Verification items for the finished model (mm, model axes). A direction names the side the tool comes from. Coordinates: 2 decimals unless noted, no trailing zeros. Loops run counter-clockwise (first coordinate to the right, second up) from the corner with the lowest first, then second, coordinate; pieces in that order, holes last.
Q1. Access from +Z, -Z, +X, -X, +Y, -Y to the whole of each face (thin tool, end or side, straight path). Record for faces 1 (the face through (-19.96, 11.57, 17)), 2 (the face through (12.5, 3, 0)).
Q2. Sectioned sample at C-C (y = 42.5). Enter the section's corners in (x, z), then the cut area to 3 significant figures.
Q3. Mould release check, pull along X, two halves, no side actions. Record for faces 3 (the face through (0, 0, 0)), 4 (the face through (-17.5, 45, 0)), 5 (the face through (-22.5, 42, 0)): +X half, -X half, draft (parallel to the pull), parting line (faces both ways), or undercut.
Q4. Sectioned sample at D-D (z = 3). Enter the section's corners in (x, y), then the cut area to 3 significant figures.
Q5. Material ranges on probe 1 along Y at (x, z) = (17.5, 0); probe 2 along Z at (x, y) = (18, 4.5); probe 3 along X at (y, z) = (34.5, 11), recorded low to high.
Q6. Go/stop test with flat-tipped pins: P1, Ø1, axis at x = -15.5, z = -3, coming from the +Y side; P2, Ø2, axis at y = 3.5, z = -10, coming from the +X side; P3, Ø4, axis at y = 18, z = 12, coming from the +X side. Record where each tip stops, or that it passes through.
Q7. Sectioned sample at A-A (y = 27). Enter the section's corners in (x, z).
Q8. Sectioned sample at B-B (x = 14). Enter the section's corners in (y, z), then the cut area to 3 significant figures.
```python
from build123d import *

# Parameters (mm, degrees)
SKETCH1_W           = 45
SKETCH1_H           = 43
BOSS_EXTRUDE1_DEPTH = 6
SKETCH2_W           = 5
SKETCH2_H           = 43
BOSS_EXTRUDE2_DEPTH = 80
CUT_EXTRUDE1_REACH  = 99.254
SKETCH3_R           = 11.25
SKETCH3_R_2         = 1.5
CUT_EXTRUDE2_REACH  = 99.254
SKETCH4_R           = 4
FILLET1_R           = 20
SKETCH6_R           = 2
CUT_EXTRUDE4_DEPTH  = 10


with BuildPart() as part:
    # Sketch1 → Boss-Extrude1 (new body)
    with BuildSketch(Plane(origin=(0, 0, 0), x_dir=(1, 0, 0), z_dir=(0, 1, 0))):
        Rectangle(SKETCH1_W, SKETCH1_H)
    extrude(amount=BOSS_EXTRUDE1_DEPTH)

    # Sketch2 → Boss-Extrude2 (add)
    with BuildSketch(Plane(origin=(0, 6, 0), x_dir=(1, 0, 0), z_dir=(0, 1, 0))):
        with Locations((-20, 0)):
            Rectangle(SKETCH2_W, SKETCH2_H)
    extrude(amount=BOSS_EXTRUDE2_DEPTH)

    # Sketch3 → Cut-Extrude1 (cut, up to next)
    with BuildSketch(Plane(origin=(-17.5, 0, 0), x_dir=(0, 0, -1), z_dir=(1, 0, 0)), mode=Mode.PRIVATE) as cut_extrude1_sk1:
        with Locations((0, 27)):
            Circle(SKETCH3_R)
    cut_extrude1_tool1 = extrude(cut_extrude1_sk1.sketch, amount=-CUT_EXTRUDE1_REACH, mode=Mode.PRIVATE) & part.part
    # Sketch3 → Cut-Extrude1 (cut, up to next)
    with BuildSketch(Plane(origin=(-17.5, 0, 0), x_dir=(0, 0, -1), z_dir=(1, 0, 0)), mode=Mode.PRIVATE) as cut_extrude1_sk2:
        with Locations((-15.5, 42.5)):
            Circle(SKETCH3_R_2)
    cut_extrude1_tool2 = extrude(cut_extrude1_sk2.sketch, amount=-CUT_EXTRUDE1_REACH, mode=Mode.PRIVATE) & part.part
    # Sketch3 → Cut-Extrude1 (cut, up to next)
    with BuildSketch(Plane(origin=(-17.5, 0, 0), x_dir=(0, 0, -1), z_dir=(1, 0, 0)), mode=Mode.PRIVATE) as cut_extrude1_sk3:
        with Locations((15.5, 42.5)):
            Circle(SKETCH3_R_2)
    cut_extrude1_tool3 = extrude(cut_extrude1_sk3.sketch, amount=-CUT_EXTRUDE1_REACH, mode=Mode.PRIVATE) & part.part
    # Sketch3 → Cut-Extrude1 (cut, up to next)
    with BuildSketch(Plane(origin=(-17.5, 0, 0), x_dir=(0, 0, -1), z_dir=(1, 0, 0)), mode=Mode.PRIVATE) as cut_extrude1_sk4:
        with Locations((15.5, 11.5)):
            Circle(SKETCH3_R_2)
    cut_extrude1_tool4 = extrude(cut_extrude1_sk4.sketch, amount=-CUT_EXTRUDE1_REACH, mode=Mode.PRIVATE) & part.part
    # Sketch3 → Cut-Extrude1 (cut, up to next)
    with BuildSketch(Plane(origin=(-17.5, 0, 0), x_dir=(0, 0, -1), z_dir=(1, 0, 0)), mode=Mode.PRIVATE) as cut_extrude1_sk5:
        with Locations((-15.5, 11.5)):
            Circle(SKETCH3_R_2)
    cut_extrude1_tool5 = extrude(cut_extrude1_sk5.sketch, amount=-CUT_EXTRUDE1_REACH, mode=Mode.PRIVATE) & part.part
    add(cut_extrude1_tool1.solids().sort_by_distance((-17.5, 27, 0))[0], mode=Mode.SUBTRACT)
    add(cut_extrude1_tool2.solids().sort_by_distance((-17.5, 42.5, 15.5))[0], mode=Mode.SUBTRACT)
    add(cut_extrude1_tool3.solids().sort_by_distance((-17.5, 42.5, -15.5))[0], mode=Mode.SUBTRACT)
    add(cut_extrude1_tool4.solids().sort_by_distance((-17.5, 11.5, -15.5))[0], mode=Mode.SUBTRACT)
    add(cut_extrude1_tool5.solids().sort_by_distance((-17.5, 11.5, 15.5))[0], mode=Mode.SUBTRACT)

    # Sketch4 → Cut-Extrude2 (cut, up to next)
    with BuildSketch(Plane(origin=(-17.5, 0, 0), x_dir=(0, 0, -1), z_dir=(1, 0, 0)), mode=Mode.PRIVATE) as cut_extrude2_sk1:
        with Locations((0, 69)):
            Circle(SKETCH4_R)
    cut_extrude2_tool1 = extrude(cut_extrude2_sk1.sketch, amount=-CUT_EXTRUDE2_REACH, mode=Mode.PRIVATE) & part.part
    add(cut_extrude2_tool1.solids().sort_by_distance((-17.5, 69, 0))[0], mode=Mode.SUBTRACT)

    # Fillet1
    fillet1_edges = [part.edges().sort_by_distance(p)[0] for p in [
        (-20, 86, -21.5),
        (-20, 86, 21.5),
    ]]
    fillet(fillet1_edges, radius=FILLET1_R)

    # Sketch6 → Cut-Extrude4 (cut)
    with BuildSketch(Plane(origin=(22.5, 0, 0), x_dir=(0, 0, -1), z_dir=(1, 0, 0))):
        with Locations((0, 3)):
            Circle(SKETCH6_R)
        with Locations((10, 3)):
            Circle(SKETCH6_R)
        with Locations((-10, 3)):
            Circle(SKETCH6_R)
    extrude(amount=-CUT_EXTRUDE4_DEPTH, mode=Mode.SUBTRACT)


solid = part.part
```
Geometry check:
1. face 1: +X, -X
1. face 2: +X
2. outline: (-22.5, -21.5) - (-17.5, -21.5) - (-17.5, -17) - (-22.5, -17) - close; (-22.5, -14) - (-17.5, -14) - (-17.5, 14) - (-22.5, 14) - close; (-22.5, 17) - (-17.5, 17) - (-17.5, 21.5) - (-22.5, 21.5) - close
2. area: 185 mm2
3. face 3: draft
3. face 4: +X half
3. face 5: -X half
4. outline: (-22.5, 0) - (22.5, 0) - (22.5, 6) - (-17.5, 6) - (-17.5, 16.16) - (-22.5, 16.16) - close; (-22.5, 37.84) - (-17.5, 37.84) - (-17.5, 66.35) - (-22.5, 66.35) - close; (-22.5, 71.65) - (-17.5, 71.65) - (-17.5, 85.94) - (-22.5, 85.94) - close
4. area: 535 mm2
5. probe 1: y = 0 to 1, 5 to 6
5. probe 2: z = -21.5 to -11.32, -8.68 to -1.32, 1.32 to 8.68, 11.32 to 21.5
5. probe 3: x = -22.5 to -17.5
6. P1: stops at y = 6
6. P2: stops at x = 12.5
6. P3: stops at x = -17.5
7. outline: (-22.5, -21.5) - (-17.5, -21.5) - (-17.5, -11.25) - (-22.5, -11.25) - close; (-22.5, 11.25) - (-17.5, 11.25) - (-17.5, 21.5) - (-22.5, 21.5) - close
8. outline: (0, -21.5) - (6, -21.5) - (6, 21.5) - (0, 21.5) - close; hole circle Ø4 at (3, -10); hole circle Ø4 at (3, 0); hole circle Ø4 at (3, 10)
8. area: 220 mm2
